Geometry: see drawing. Coordinates: mm, zero at the bounding-box minimum. Round coordinates to 2 decimals unless told otherwise and drop trailing zeros. Loops run counter-clockwise (first coordinate to the right, second up) from the corner with the lowest first, then second, coordinate; pieces in that order, holes last. Notation, with made-up numbers: (-22, 20) - (-7, 20) arc R25 cw to (-7, 56) - close; hole circle Ø8 at (-1, 59.5). An arc over 180 degrees is marked (long way). Write item = value, one per line. Start each with the question number.
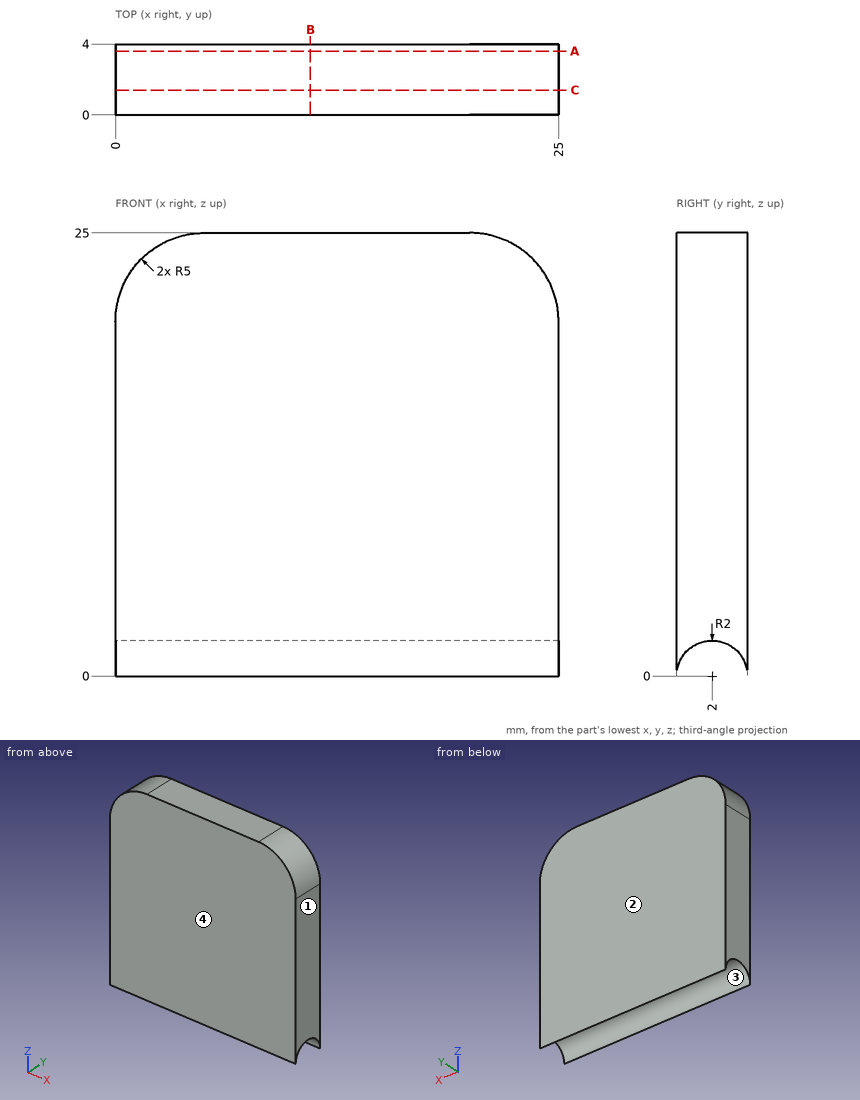
(1) Cut plane C-C (y = 1.4). Output: boundary loops of the cut face in (x, z).
(2) Cut plane B-B (x = 11). Output: boundary loops of the cut face in (y, z), and give its area (3 significant figures).
(3) Cut plane A-A (y = 3.6). Output: boundary loops of the cut face in (x, z), and give its area (3 significant figures).
(4) Mould query, pull axis Y, two halves, no side actions, for the marked faces 1, 2, 3 and 4. Classes: +Y half, -Y half, draft (parallel to the pull), parting line (faces both ways), or undercut.
(5) Material intervals for line 1 along Z through (x, y) = (7, 2.05); line 2 along Z through (x, y) = (11, 2.6); line 3 along X through (y, z) = (1.15, 21.5), sorted ascending. Write a range as from..to.
Solution:
q1.outline = (0, 1.91) - (25, 1.91) - (25, 20) arc R5 ccw to (20, 25) - (5, 25) arc R5 ccw to (0, 20) - close
q2.outline = (0, 0) arc R2 cw to (4, 0) - (4, 25) - (0, 25) - close
q2.area = 93.7 mm^2
q3.outline = (0, 1.2) - (25, 1.2) - (25, 20) arc R5 ccw to (20, 25) - (5, 25) arc R5 ccw to (0, 20) - close
q3.area = 584 mm^2
q4.face_1 = draft
q4.face_2 = +Y half
q4.face_3 = undercut
q4.face_4 = -Y half
q5.line_1 = 2..25
q5.line_2 = 1.91..25
q5.line_3 = 0.23..24.77
